Autodesk Inventor part; units mm, degrees
ref_plane "YZ Plane" through (0, 0, 0) normal (1, 0, 0) x (0, 1, 0)
ref_plane "XZ Plane" through (0, 0, 0) normal (0, 1, 0) x (-1, 0, 0)
ref_plane "XY Plane" through (0, 0, 0) normal (0, 0, 1) x (1, 0, 0)
sketch "Sketch1" plane through (0, 0, 0) normal (0, 1, 0) x (-1, 0, 0)
  line L0 (0, 0) -> (-110, 0)
  line L1 (-110, 0) -> (-110, -90)
  line L2 (-110, -90) -> (0, -90)
  line L3 (0, -90) -> (0, 0)
  line L4 (0, -90) -> (-11.075, -90)
  line L5 (-11.075, -90) -> (-11.075, 0) construction
  line L6 (-11.075, 0) -> (0, 0)
  line L7 (0, 0) -> (0, -90)
  line L8 (-110, -90) -> (-98.925, -90)
  line L9 (-98.925, -90) -> (-98.925, 0) construction
  line L10 (-98.925, 0) -> (-110, 0)
  line L11 (-110, 0) -> (-110, -90)
  line L12 (-11.075, -90) -> (-11.075, -84)
  circle A0 centre (-11.075, -80.425) radius 3.575
  line L13 (-11.075, -76.85) -> (-11.075, -16.85) construction
  circle A1 centre (-11.075, -13.275) radius 3.575
  line L14 (-98.925, -90) -> (-98.925, -84)
  circle A2 centre (-98.925, -80.425) radius 3.575
  line L15 (-98.925, -76.85) -> (-98.925, -16.85) construction
  circle A3 centre (-98.925, -13.275) radius 3.575
  line L16 (-55, 0) -> (-55, -45)
  circle A4 centre (-55, -45) radius 15
  circle A5 centre (-55, -45) radius 25
  circle A6 centre (-55, -70) radius 3.25
  circle A7 centre (-33.3494, -32.5) radius 3.25
  circle A8 centre (-76.6506, -32.5) radius 3.25
  dimension "d7" = 7.15
  dimension "d11" = 7.15
  dimension "d15" = 50
  dimension "d0" = 90
  dimension "d1" = 110
  dimension "d2" = 11.075
  dimension "d3" = 11.075
  dimension "d4" = 6
  dimension "d5" = 7.15
  dimension "d6" = 60
  dimension "d8" = 6
  dimension "d9" = 7.15
  dimension "d10" = 60
  dimension "d12" = 55
  dimension "d13" = 45
  dimension "d14" = 30
  dimension "d16" = 6.5
  dimension "d19" = 360
  dimension "d37" = 87.85
extrude "Extrusion1" add sketch "Sketch1" along normal blind 5 contours A5 A7 A6 A8 | A2 | A0 | L3 L2 L1 L0 | A7 A5 | A5 A7 | A8 A5 | A5 A8 | A6 A5 | A5 A6 | A1 | A3
hole "Hole1" at (98.925, 0, -80.425) at (11.075, 0, -80.425) at (11.075, 0, -13.275) at (98.925, 0, -13.275) direction (0, 1, 0) diameter 8 depth 10
hole "Hole2" at (55, 0, -70) at (76.6506, 0, -32.5) at (33.3494, 0, -32.5) direction (0, 1, 0) diameter 8 depth 10
properties part number "motorbracket2"
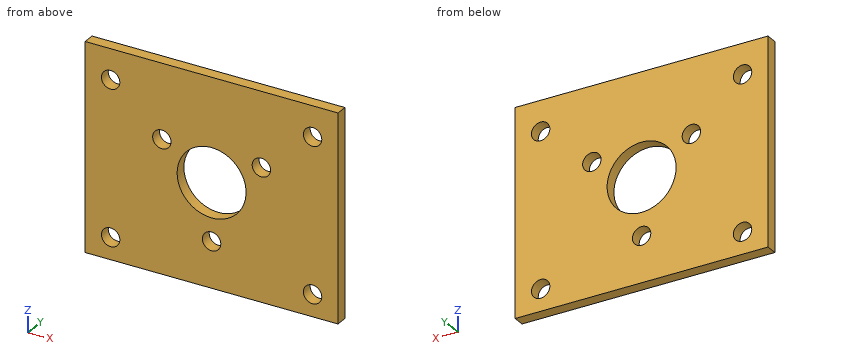
Part model, mm, in its own coordinate system. Give positions to 0.01 mm unless a question says otherwise; leave off trailing zeros. Write each loop counter-clockwise with the first axis right and the second up, starting at its lowest first coordinate (ties: lowest second). Pieces come first, ordered by that corner, then holes. Notation, with made-up numbers: (-7, 6.25) -> (14, 6.25) arc R20 cw to (14, 38.25) -> close; hole circle Ø3 at (43, 26.5). An arc over 180 degrees is marked (long way). Put each result on its own line as item: value. Start each with the question number.
Item 1: Cut at C-C (z = -45). List the corners of the cut face in (x, y), then the cut area to 3 significant figures.
Item 2: Wall check: L1, parallel to Z at x = 55, y = 1.5; L2, parallel to Z at x = 11, y = 0.8; L3, parallel to X at y = 3.8, z = -29.5. Give the ranges that are in metal, low to high. Write a range as [from, to].
Item 3: Cut at D-D (y = 4). State how many separate pieces and enclosed holes the cut face has, then the cut area to 3 significant figures.
Item 4: Cut at A-A (x = 55). List the corners of the cut face in (y, z), then the cut area to 3 significant figures.
Item 5: Cut at B-B (z = -70). List the corners of the cut face in (x, y).
Item 6: Pin check, flat tip, straight feed: pin 1 Ø13 at (x, z) = (98.925, -13.275) entering from +Y. Stop position of the tip, or through.
Answer list:
1. outline: (0, 0) -> (40, 0) -> (40, 5) -> (0, 5) -> close; (70, 0) -> (110, 0) -> (110, 5) -> (70, 5) -> close
1. area: 400 mm2
2. L1: z = [-90, -74], [-66, -60], [-30, 0]
2. L2: z = [-90, -84.42], [-76.43, -17.27], [-9.28, 0]
2. L3: x = [0, 30.7], [36, 74], [79.3, 110]
3. separate pieces: 1
3. enclosed holes: 8
3. area: 8,840 mm2
4. outline: (0, -90) -> (5, -90) -> (5, -74) -> (0, -74) -> close; (0, -66) -> (5, -66) -> (5, -60) -> (0, -60) -> close; (0, -30) -> (5, -30) -> (5, 0) -> (0, 0) -> close
4. area: 260 mm2
5. outline: (0, 0) -> (51, 0) -> (51, 5) -> (0, 5) -> close; (59, 0) -> (110, 0) -> (110, 5) -> (59, 5) -> close
6. pin 1: stops at y = 5
